Verification items for this drawing (mm, ordinates from the low corner). A direction names the side the tool comes from. Coordinates: 2 decimals unless noted, no trailing zeros. Loops run counter-clockwise (first coordinate to the right, second up) from the corner with the lowest first, then second, coordinate; pieces in that order, holes last. Notation, with made-up numbers: M 23,47 L 35,47 A15 ccw 35,61 Z; hole C -28,46.25 d10. An arc over 180 degrees is marked long. Use CSV: the item, a comma, the result in double quotes.
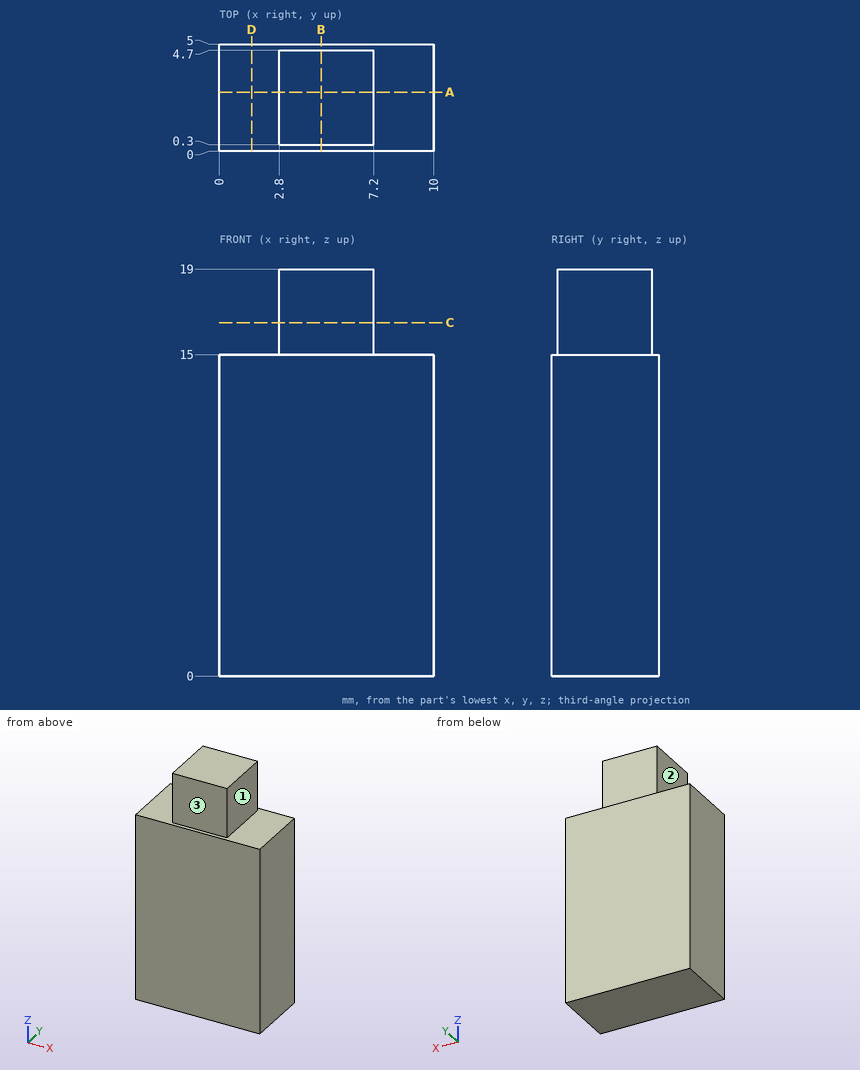
1. Thickness scan on line 1 (Z direction, x = 2.5, y = 0.7); line 2 (X direction, y = 4.2, z = 16). Record the ranges inside material, lowest first. Write a range as [from, to].
The answers:
line 1,"[0, 15]"
line 2,"[2.8, 7.2]"
2. Section check C-C, the plane z = 16.5. Record the cut outline in (x, y), plus the area to 3 significant figures.
The answers:
outline,"M 2.8,0.3 L 7.2,0.3 L 7.2,4.7 L 2.8,4.7 Z"
area,"19.4 mm^2"
3. Section check B-B, the plane x = 4.75. Record the cut outline in (y, z), plus the area to 3 significant figures.
The answers:
outline,"M 0,0 L 5,0 L 5,15 L 4.7,15 L 4.7,19 L 0.3,19 L 0.3,15 L 0,15 Z"
area,"92.6 mm^2"
4. Section check D-D, the plane x = 1.5. Record the cut outline in (y, z).
The answers:
outline,"M 0,0 L 5,0 L 5,15 L 0,15 Z"
5. Set-up check for the marked faces 1, 2 and 3: record each of +Z, -Z, +X, -X, +Y, -Y from which the full face is reachable in a straight line by a thin tool's end or side.
The answers:
face 1,"+Z, +X, +Y, -Y"
face 2,"+Z, -X, +Y, -Y"
face 3,"+Z, +X, -X, -Y"
6. Gauge pin test, flat ends, axial feed: P1, Ø2, axis at y = 1.5, z = 17.5, coming from the -X side; P2, Ø2, axis at x = 5.5, z = 17, coming from the +Y side; P3, Ø3, axis at x = 5, z = 17, coming from the -Y side. Record the tip position at first contact, or that the pin passes through.
The answers:
P1,"x = 2.8"
P2,"y = 4.7"
P3,"y = 0.3"
7. Section check A-A, the plane y = 2.75. Record the cut outline in (x, z), plus the area to 3 significant figures.
The answers:
outline,"M 0,0 L 10,0 L 10,15 L 7.2,15 L 7.2,19 L 2.8,19 L 2.8,15 L 0,15 Z"
area,"168 mm^2"
